CAD build for the part. Positions are in the model's coordinates, mm. A direction names the side the tool comes from. Give positions to 0.01 mm unless a question says otherwise; leave off trailing zeros. Write each loop counter-clockwise with the first axis right and the second up, starting at its lowest first coordinate (ties: lowest second). Pieces come first, ordered by that corner, then holes. Notation, with made-up numbers: (48.25, -2.5) - (72.25, -2.5) arc R27 cw to (72.25, 24.5) - close; hole circle Ø6 at (41, 20.5). An arc over 180 degrees is marked (long way). Write item = value, one per line. Start each with the question number.
```python
from build123d import *

# Parameters (mm, degrees)
SKETCH1_R           = 3.535533906
BOSS_EXTRUDE1_DEPTH = 6.5
SKETCH1_6_W         = 3.5
SKETCH1_6_H         = 3.5
BOSS_EXTRUDE2_DEPTH = 4
SKETCH4_R           = 4.25
BOSS_EXTRUDE5_DEPTH = 15
SKETCH2_R           = 2.5
BOSS_EXTRUDE3_DEPTH = 3.2
SKETCH3_R           = 1.5
BOSS_EXTRUDE4_DEPTH = 1.8
BOSS_EXTRUDE6_DEPTH = 15
CHAMFER1_SIZE       = 0.25


with BuildPart() as part:
    # Sketch1 → Boss-Extrude1 (new body)
    with BuildSketch(Plane(origin=(0, 0, 0), x_dir=(1, 0, 0), z_dir=(0, 1, 0))):
        with Locations(Location((0, 0, 0), (0, 0, 270))):
            Circle(SKETCH1_R)
    extrude(amount=-BOSS_EXTRUDE1_DEPTH)

    # Sketch1<6> → Boss-Extrude2 (add)
    with BuildSketch(Plane(origin=(0, 0, 0), x_dir=(1, 0, 0), z_dir=(0, 1, 0))):
        Rectangle(SKETCH1_6_W, SKETCH1_6_H)
    extrude(amount=BOSS_EXTRUDE2_DEPTH)

    # Sketch4 → Boss-Extrude5 (add)
    with BuildSketch(Plane.XZ.offset(6.5)):
        with Locations(Location((0, 0, 0), (0, 0, 270))):
            Circle(SKETCH4_R)
    extrude(amount=BOSS_EXTRUDE5_DEPTH)

    # Sketch2 → Boss-Extrude3 (add)
    with BuildSketch(Plane.XZ.offset(21.5)):
        with Locations(Location((0, 0, 0), (0, 0, 270))):
            Circle(SKETCH2_R)
    extrude(amount=BOSS_EXTRUDE3_DEPTH)

    # Sketch3 → Boss-Extrude4 (add)
    with BuildSketch(Plane.XZ.offset(24.7)):
        with Locations(Location((0, 0, 0), (0, 0, 270))):
            Circle(SKETCH3_R)
    extrude(amount=BOSS_EXTRUDE4_DEPTH)

    # Sketch5 → Boss-Extrude6 (add)
    with BuildSketch(Plane(origin=(0, -6.5, 0), x_dir=(1, 0, 0), z_dir=(0, 1, 0))):
        with BuildLine():
            Line((-9.330348818, 12.159547317), (-1.19003001, 1.550877304))
            ThreePointArc((-1.19003001, 1.550877304), (0, 0.964019448), (1.19003001, 1.550877304))
            Line((1.19003001, 1.550877304), (9.330348818, 12.159547317))
            ThreePointArc((9.330348818, 12.159547317), (9.616170653, 13.340759097), (8.933207003, 14.346003368))
            ThreePointArc((8.933207003, 14.346003368), (0, 16.9), (-8.933207003, 14.346003368))
            ThreePointArc((-8.933207003, 14.346003368), (-9.616170653, 13.340759097), (-9.330348818, 12.159547317))
        make_face()
        with BuildLine():
            Line((12.159547317, 9.330348818), (1.550877304, 1.19003001))
            ThreePointArc((1.550877304, 1.19003001), (0.964019448, 0), (1.550877304, -1.19003001))
            Line((1.550877304, -1.19003001), (12.159547317, -9.330348818))
            ThreePointArc((12.159547317, -9.330348818), (13.340759097, -9.616170653), (14.346003368, -8.933207003))
            ThreePointArc((14.346003368, -8.933207003), (16.9, 0), (14.346003368, 8.933207003))
            ThreePointArc((14.346003368, 8.933207003), (13.340759097, 9.616170653), (12.159547317, 9.330348818))
        make_face()
        with BuildLine():
            Line((9.330348818, -12.159547317), (1.19003001, -1.550877304))
            ThreePointArc((1.19003001, -1.550877304), (0, -0.964019448), (-1.19003001, -1.550877304))
            Line((-1.19003001, -1.550877304), (-9.330348818, -12.159547317))
            ThreePointArc((-9.330348818, -12.159547317), (-9.616170653, -13.340759097), (-8.933207003, -14.346003368))
            ThreePointArc((-8.933207003, -14.346003368), (0, -16.9), (8.933207003, -14.346003368))
            ThreePointArc((8.933207003, -14.346003368), (9.616170653, -13.340759097), (9.330348818, -12.159547317))
        make_face()
        with BuildLine():
            Line((-12.159547317, -9.330348818), (-1.550877304, -1.19003001))
            ThreePointArc((-1.550877304, -1.19003001), (-0.964019448, 0), (-1.550877304, 1.19003001))
            Line((-1.550877304, 1.19003001), (-12.159547317, 9.330348818))
            ThreePointArc((-12.159547317, 9.330348818), (-13.340759097, 9.616170653), (-14.346003368, 8.933207003))
            ThreePointArc((-14.346003368, 8.933207003), (-16.9, 0), (-14.346003368, -8.933207003))
            ThreePointArc((-14.346003368, -8.933207003), (-13.340759097, -9.616170653), (-12.159547317, -9.330348818))
        make_face()
    extrude(amount=-BOSS_EXTRUDE6_DEPTH)

    # Chamfer1
    chamfer1_edges = [part.edges().sort_by_distance(p)[0] for p in [
        (0, -6.5, -3.535533906),
        (0, 0, -3.535533906),
        (0, -21.5, 2.5),
        (0, -24.7, 2.5),
        (0, -24.7, 1.5),
        (0, -26.5, 1.5),
        (1.75, 4, 0),
        (0, 4, -1.75),
        (-1.75, 4, 0),
        (0, 4, 1.75),
    ]]
    chamfer(chamfer1_edges, length=CHAMFER1_SIZE)


solid = part.part
```
1. Wall check: line 1 along Z through (x, y) = (5, -19); line 2 along Y through (x, z) = (-8.5, 14.5); line 3 along X through (y, z) = (-9, 4.5). Give the ranges that are in metal, low to high.
2. Tool access for faces 1 (the flat face through (-5.91, -13.9, 7.7)), 2 (the flat face through (0, 2, -1.75)), 3 (the flat face through (-2, -24.7, 0)): list every direction of +Z, -Z, +X, -X, +Y, -Y with a clear straight run to the whole face (end or side of a thin tool).
3. Cut at A-A (z = -4.5). Give the cut face in (x, y).
4. Pin check, flat tips, straight feed: pin 1 Ø2 at (x, y) = (13.5, -17) entering from +Z; pin 2 Ø8 at (x, z) = (-4, 12) entering from +Y; pin 3 Ø8 at (x, z) = (-1, 8.5) entering from -Y; pin 4 Ø12 at (x, y) = (-12, 0.5) entering from -Z. Stop position of each tip, or through.
5. Cut at B-B (y = -11.5). Give the cut face in (x, z), then the cut area to 3 significant figures.
6. Mould opens along Z. For faces 4 (the flat face through (7.83, -13.9, -6.01)), 5 (the cylindrical face through (-3.45, -3.21, -0.77)), 6 (the flat face through (-7.7, -13.9, -5.91)), 7 (the flat face through (1.75, 2, 0)) say: +Z half, -Z half, draft (parallel to the pull), parting line (faces both ways), or undercut.
Output:
q1.line_1 = -16.14 to -6.52, -3.84 to 3.84, 6.52 to 16.14
q1.line_2 = -21.5 to -6.5
q1.line_3 = -16.29 to -5.86, -3.45 to 3.45, 5.86 to 16.29
q2.face_1 = +Y, -Y
q2.face_2 = -Z, +X, -X, +Y
q2.face_3 = -Y
q3.outline = (-16.29, -21.5) - (-5.86, -21.5) - (-5.86, -6.5) - (-16.29, -6.5) - close; (-3.45, -21.5) - (3.45, -21.5) - (3.45, -6.5) - (-3.45, -6.5) - close; (5.86, -21.5) - (16.29, -21.5) - (16.29, -6.5) - (5.86, -6.5) - close
q4.pin_1 = 9.64
q4.pin_2 = -6.5
q4.pin_3 = -21.5
q4.pin_4 = through
q5.outline = (-14.35, -8.93) arc R1.5 ccw to (-12.16, -9.33) - (-3.37, -2.59) arc R4.25 ccw to (-2.59, -3.37) - (-9.33, -12.16) arc R1.5 ccw to (-8.93, -14.35) arc R16.9 ccw to (8.93, -14.35) arc R1.5 ccw to (9.33, -12.16) - (2.59, -3.37) arc R4.25 ccw to (3.37, -2.59) - (12.16, -9.33) arc R1.5 ccw to (14.35, -8.93) arc R16.9 ccw to (14.35, 8.93) arc R1.5 ccw to (12.16, 9.33) - (3.37, 2.59) arc R4.25 ccw to (2.59, 3.37) - (9.33, 12.16) arc R1.5 ccw to (8.93, 14.35) arc R16.9 ccw to (-8.93, 14.35) arc R1.5 ccw to (-9.33, 12.16) - (-2.59, 3.37) arc R4.25 ccw to (-3.37, 2.59) - (-12.16, 9.33) arc R1.5 ccw to (-14.35, 8.93) arc R16.9 ccw to start
q5.area = 753 mm2
q6.face_4 = undercut
q6.face_5 = parting line
q6.face_6 = undercut
q6.face_7 = draft
